Here's how the part is built. I have some questions about the finished solid (model axes, mm). Face numbers are marked on the shaded views. A direction names the side the tool comes from. Coordinates: 2 decimals unless noted, no trailing zeros. Loops run counter-clockwise (first coordinate to the right, second up) from the corner with the lowest first, then second, coordinate; pieces in that order, holes last. Notation, with made-up numbers: (77, 84.5) - (124, 84.5) arc R24 cw to (124, 121.5) - close; hole circle Ø5 at (12.5, -7). An arc over 180 degrees is marked (long way). Use a Markdown table: item, result.
```python
from build123d import *

# Parameters (mm, degrees)
F1_DEPTH      = 11.1125
F2_R          = 3.175
F2_R_2        = 1.5875
F2_R_3        = 2.15265
F3_DEPTH      = 8.73125
F4_R          = 2.38125
F5_DEPTH      = 1.5875
F6_R          = 3.96875
F6_R_2        = 3.175
F7_DEPTH      = 0.79375
F7_DEPTH_BACK = 5.55625
F8_R          = 5.55624
F10_R         = 3.96875
F11_DEPTH     = 5.55625
F12_C1_SIZE   = 2.38125
F12_C2_SIZE   = 2.38125
F12_C3_SIZE   = 2.38125


# Not quite as in the source:
# - a fillet or chamfer is up to 0.001 mm smaller than in the source, because OpenCascade refuses the exact size


with BuildPart() as f1:
    # F0 (on Top) → F1 (new body)
    with BuildSketch(Plane.XY):
        Polygon((-12.7, 0), (0, 0), (0, -6.35), (11.1125, -6.35), (11.1125, 0), (26.9875, 0), (26.9875, -6.35), (38.1, -6.35), (38.1, -3.571875), (50.8, -3.571875), (50.8, 1.5875), (38.1, 1.5875), (38.1, 2.38125), (-12.7, 2.38125), align=None)
    extrude(amount=F1_DEPTH)

    # F2 (on face) → F3 (cut, through all)
    with BuildSketch(Plane(origin=(0, 2.38125, 0), x_dir=(-1, 0, 0), z_dir=(0, 1, 0))):
        with Locations((-45.24375, 5.55625)):
            Circle(F2_R)
        with Locations((7.14375, 5.55625)):
            Circle(F2_R_2)
        with Locations((-5.55625, 5.55625)):
            Circle(F2_R_3)
        with Locations((-32.54375, 5.55625)):
            Circle(F2_R_3)
    extrude(amount=-F3_DEPTH, mode=Mode.SUBTRACT)

    # F4 (on face) → F5 (cut)
    with BuildSketch(Plane.XZ):
        with Locations((-7.14375, 5.55625)):
            Circle(F4_R)
    extrude(amount=-F5_DEPTH, mode=Mode.SUBTRACT)

    # F6 (on face) → F7 (join, two sides)
    with BuildSketch(Plane(origin=(0, 1.5875, 0), x_dir=(-1, 0, 0), z_dir=(0, 1, 0))) as f7_sk:
        with Locations((-45.24375, 5.55625)):
            Circle(F6_R)
        with Locations((-45.24375, 5.55625)):
            Circle(F6_R_2, mode=Mode.SUBTRACT)
    extrude(amount=F7_DEPTH)
    extrude(f7_sk.sketch, amount=-F7_DEPTH_BACK)

    # F8 (radius 5.55625 in the source; OpenCascade refuses exactly that, so slightly less here)
    f8_edges = [f1.edges().sort_by_distance(p)[0] for p in [
        (0, -3.175, 0),
        (0, -3.175, 11.1125),
        (38.1, -4.960938, 0),
        (38.1, -4.960938, 11.1125),
        (38.1, 1.984375, 0),
        (38.1, 1.984375, 11.1125),
        (11.1125, -3.175, 11.1125),
        (11.1125, -3.175, 0),
        (26.9875, -3.175, 11.1125),
        (26.9875, -3.175, 0),
        (50.8, -0.992188, 11.1125),
        (50.8, -0.992188, 0),
        (-12.7, 1.190625, 11.1125),
        (-12.7, 1.190625, 0),
    ]]
    fillet(f8_edges, radius=F8_R)

    # F10 (on face) → F11 (cut, through all)
    with BuildSketch(Plane(origin=(0, 2.38125, 0), x_dir=(-1, 0, 0), z_dir=(0, 1, 0))):
        with Locations((-32.54375, 5.55625)):
            Circle(F10_R)
        with Locations((-5.55625, 5.55625)):
            Circle(F10_R)
    extrude(amount=-F11_DEPTH, mode=Mode.SUBTRACT)

    # F12: chamfer of 2.38125 on 5 edges, made by hand

    # F12_c1
    f12_c1_edges = [f1.edges().sort_by_distance(p)[0] for p in [
        (1.6273850181, 0, 9.4851149819),
        (0, 0, 5.55625),
        (1.6273850181, 0, 1.6273850181),
    ]]
    chamfer(f12_c1_edges, length=F12_C1_SIZE)

    # F12_c2
    f12_c2_edges = [f1.edges().sort_by_distance(p)[0] for p in [
        (28.6148850181, 0, 9.4851149819),
        (26.9875, 0, 5.55625),
        (28.6148850181, 0, 1.6273850181),
    ]]
    chamfer(f12_c2_edges, length=F12_C2_SIZE)

    # F12_c3
    f12_c3_edges = [f1.edges().sort_by_distance(p)[0] for p in [
        (11.1125, 0, 5.55625),
        (9.4851149819, 0, 9.4851149819),
        (9.4851149819, 0, 1.6273850181),
    ]]
    chamfer(f12_c3_edges, length=F12_C3_SIZE)


solid = f1.part
```
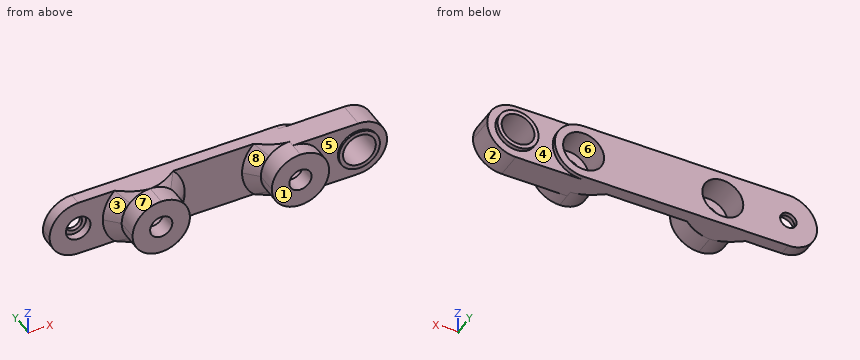
Q1. Will these pins go through, and if not, where does the flat tip stop? P1, Ø2.5, axis at x = 6.5, z = 7.5, coming from the +Y side (3 decimals); P2, Ø2.5, axis at x = 32.54, z = 5.56, coming from the -Y side; P3, Ø4, axis at x = -7.14, z = 5.56, coming from the -Y side; P4, Ø1, axis at x = 22.5, z = 2, coming from the -Y side.
Check values:
| item | result |
|---|---|
| P1 | y = -3.175 |
| P2 | through |
| P3 | y = 1.59 |
| P4 | y = 0 |
Q2. I want a section at A-A, the plane y = 1. Give the number of separate pieces and of enclosed holes in the cut face, then the cut area to 3 significant figures.
Check values:
| item | result |
|---|---|
| separate pieces | 1 |
| enclosed holes | 4 |
| area | 531 mm^2 |
Q3. If we mould it in two halves opening along X, with no side actions, what happens to the marked faces 1, 2, 3 and 4? For each: pulls with the +X half, pulls with the -X half, needs draft (parallel to the pull), parting line crosses it, or undercut.
Check values:
| item | result |
|---|---|
| face 1 | needs draft |
| face 2 | pulls with the +X half |
| face 3 | pulls with the -X half |
| face 4 | undercut |
Q4. Which directions (+Z, -Z, +X, -X, +Y, -Y) give clear straight access to the entire face, cutting with the end or side of a thin tool? Please do the marked faces 5, 6, 7 and 8.
Check values:
| item | result |
|---|---|
| face 5 | -Y |
| face 6 | +Y |
| face 7 | +Z, -X, -Y |
| face 8 | +Z, -Y |
Q5. Please list where these lines run through material, in increasing order: L1, parallel to X at y = 1.5, z = 7.5; L2, parallel to X at y = -2, z = 5.5; L3, parallel to Y at x = 16, z = 9. Write a range as from..to.
Check values:
| item | result |
|---|---|
| L1 | -12.35..-8.52, -5.77..2.1, 9.02..29.08, 36..42.73, 47.75..50.45 |
| L2 | -0.38..1.59, 9.52..11.49, 26.61..28.58, 36.51..42.07, 48.42..50.8 |
| L3 | 0..2.38 |
Q6. I want a section at B-B, the plane x = 44.5. Write out the boundary of the cut face in (y, z).
Check values:
| item | result |
|---|---|
| outline | (-3.97, 1.66) - (-3.57, 1.66) - (-3.57, 0) - (1.59, 0) - (1.59, 1.66) - (2.38, 1.66) - (2.38, 2.47) - (-3.97, 2.47) - close; (-3.97, 8.64) - (2.38, 8.64) - (2.38, 9.45) - (1.59, 9.45) - (1.59, 11.11) - (-3.57, 11.11) - (-3.57, 9.45) - (-3.97, 9.45) - close |
